Could you check a few things on this model? Use its own coordinates, in mm. Face numbers are marked on the shaded views. A direction names the side the tool comes from. Round coordinates to 2 decimals unless told otherwise and drop trailing zeros. Write each loop counter-clockwise with the first axis right and the second up, starting at its lowest first coordinate (ties: lowest second). Pieces come first, ordered by that corner, then holes. Notation, with made-up numbers: (31, 18) -> (80, 18) arc R23 cw to (80, 35) -> close; hole circle Ø10 at (32, 73.25). An arc over 180 degrees is marked (long way). Answer in a Markdown table with one row per item.
from build123d import *

# Parameters (mm, degrees)
SKETCH1_R           = 1.7
BOSS_EXTRUDE1_DEPTH = 8
CUT_EXTRUDE1_DEPTH  = 5.6
FILLET1_R           = 0.5
SKETCH5_R           = 3.7
CUT_EXTRUDE2_DEPTH  = 1
CHAMFER1_SIZE       = 2
SKETCH6_R           = 1.7
BOSS_EXTRUDE2_DEPTH = 0.4
BOSS_EXTRUDE3_START = -0.4
SKETCH7_R           = 3.7
BOSS_EXTRUDE3_DEPTH = 0.4


with BuildPart() as part:
    # Sketch1 → Boss-Extrude1 (new body)
    with BuildSketch(Plane.XY):
        with BuildLine():
            Line((0, 0), (0, 30))
            Line((0, 30), (30, 0))
            Line((30, 0), (18, 0))
            add(Edge.make_bspline(
                [(18, 0), (13.851240238, 0), (12.090763012, -2.133887147), (8.457514689, -5.611868239)],
                knots=[0, 0, 0, 0, 1, 1, 1, 1], degree=3))
            ThreePointArc((8.457514689, -5.611868239), (3.036275661, -6.598237349), (0, -2))
            Line((0, -2), (0, 0))
        make_face()
        with Locations((5, -2)):
            Circle(SKETCH1_R, mode=Mode.SUBTRACT)
    extrude(amount=BOSS_EXTRUDE1_DEPTH)

    # Sketch2 → Cut-Extrude1 (cut)
    with BuildSketch(Plane.XY.offset(8)):
        Polygon((3.2, 26.8), (3.2, 3.2), (26.8, 3.2), align=None)
    extrude(amount=-CUT_EXTRUDE1_DEPTH, mode=Mode.SUBTRACT)

    # Fillet1
    fillet1_edges = [part.edges().sort_by_distance(p)[0] for p in [
        (0, 30, 4),
        (30, 0, 4),
        (3.2, 26.8, 5.2),
        (26.8, 3.2, 5.2),
        (3.2, 3.2, 5.2),
    ]]
    fillet(fillet1_edges, radius=FILLET1_R)

    # Sketch5 → Cut-Extrude2 (cut)
    with BuildSketch(Plane(origin=(0, 0, 0), x_dir=(-1, 0, 0), z_dir=(0, 0, -1))):
        with Locations((-5, -2)):
            Circle(SKETCH5_R)
    extrude(amount=-CUT_EXTRUDE2_DEPTH, mode=Mode.SUBTRACT)

    # Chamfer1
    chamfer1_edges = [part.edges().sort_by_distance(p)[0] for p in [
        (3.3, -2, 1),
    ]]
    chamfer(chamfer1_edges, length=CHAMFER1_SIZE - 0.0001)  # a hair under: the kernel refuses the full size

    # Sketch6 → Boss-Extrude2 (add)
    with BuildSketch(Plane.XY.offset(3)):
        with Locations((5, -2)):
            Circle(SKETCH6_R)
    extrude(amount=BOSS_EXTRUDE2_DEPTH)

    # Sketch7 → Boss-Extrude3 (add)
    with BuildSketch(Plane.XY.offset(1).offset(BOSS_EXTRUDE3_START)):
        with Locations(Location((5, -2, 0), (0, 0, 180))):
            Circle(SKETCH7_R)
    extrude(amount=BOSS_EXTRUDE3_DEPTH)


solid = part.part
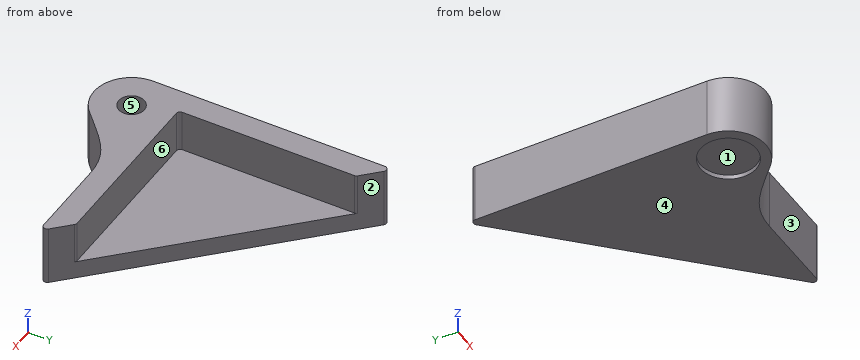
1) Please list where these lines run through material, in increasing order: line 1 (Y direction, x = 5, z = 5.25); line 2 (Z direction, x = 3.75, y = 23); line 3 (Y direction, x = 23.75, z = 3.5).
Findings:
| item | result |
|---|---|
| line 1 | y = -7 to -3.7, -0.3 to 3.2 |
| line 2 | z = 0 to 2.4 |
| line 3 | y = 0 to 3.2 |
2) For pin 1 (4 mm diameter, centred on x = 12, z = 2, fed in from +Y); pin 2 (4 mm diameter, centred on x = 25, z = 4, fed in from -Y); pin 3 (4 mm diameter, centred on x = 5, y = -2, fed in from -Z), each with a flat end and sliding along its axis, tell me the tip position at first contact or that it passes through.
Findings:
| item | result |
|---|---|
| pin 1 | stops at y = 20 |
| pin 2 | stops at y = 0 |
| pin 3 | stops at z = 0.6 |
3) Imagine slicing it at B-B, the plane y = 20. Please give me the cut outline in (x, z), plus the area to 3 significant figures.
Findings:
| item | result |
|---|---|
| outline | (0, 0) -> (10, 0) -> (10, 2.4) -> (3.2, 2.4) -> (3.2, 8) -> (0, 8) -> close |
| area | 41.9 mm^2 |
4) Imagine slicing it at C-C, the plane y = 6. Please give me the cut outline in (x, z), plus the area to 3 significant figures.
Findings:
| item | result |
|---|---|
| outline | (0, 0) -> (24, 0) -> (24, 2.4) -> (3.2, 2.4) -> (3.2, 8) -> (0, 8) -> close |
| area | 75.5 mm^2 |
5) For the marked faces 4, 5 and 6, which set-ups out of +Z, -Z, +X, -X, +Y, -Y let a thin tool reach every point of the face, with its end or its side?
Findings:
| item | result |
|---|---|
| face 4 | -Z, +X, -X, +Y, -Y |
| face 5 | +Z |
| face 6 | +Z, +X, +Y |
6) Thinking about a two-plate mould opening in X: for the marked faces 1, 2 and 3, which applies, +X half, -X half, draft (parallel to the pull), parting line (faces both ways), or undercut?
Findings:
| item | result |
|---|---|
| face 1 | undercut |
| face 2 | +X half |
| face 3 | draft |
